from build123d import *

# Parameters (mm, degrees)
F0_R     = 11
F1_DEPTH = 2
F2_R     = 2.5
F3_DEPTH = 25
F4_R     = 11
F4_R_2   = 9
F5_DEPTH = 10


with BuildPart() as f1:
    # F0 (on Front) → F1 (new body)
    with BuildSketch(Plane.XZ):
        Circle(F0_R)
    extrude(amount=F1_DEPTH)

    # F2 (on face) → F3 (cut)
    with BuildSketch(Plane.XZ.offset(2)):
        Circle(F2_R)
    extrude(amount=-F3_DEPTH, mode=Mode.SUBTRACT)

    # F4 (on face) → F5 (join)
    with BuildSketch(Plane.XZ.offset(2)):
        Circle(F4_R)
        Circle(F4_R_2, mode=Mode.SUBTRACT)
    extrude(amount=F5_DEPTH)


solid = f1.part
Source: CAD feature listing. Evaluate the final solid. Frame: model axes, mm. A direction names the side the tool comes from. Coordinates: 2 decimals unless noted, no trailing zeros. Loops run counter-clockwise (first coordinate to the right, second up) from the corner with the lowest first, then second, coordinate; pieces in that order, holes last. Notation, with made-up numbers: (65.5, -28.5) - (112.5, -28.5) arc R33 cw to (112.5, 8.5) - close; hole circle Ø6 at (-37.5, -1.5). An arc over 180 degrees is marked (long way). One line per item, written item: value. Start each with the question number.
1. Mould query, pull axis Z, two halves, no side actions, for faces 3 (the flat face through (-3, 0, 0)), 4 (the cylindrical face through (-2.38, -5.92, -10.74)), 5 (the cylindrical face through (-0.54, -1.01, -2.44)). Classes: pulls with the +Z half, pulls with the -Z half, needs draft (parallel to the pull), parting line crosses it, or undercut.
2. Contact query for flat-ended pins moving along their axis: P1, Ø2, axis at y = -7, z = -3, coming from the -X side; P2, Ø4, axis at y = -8.5, z = -3.5, coming from the +X side; P3, Ø12, axis at x = 7.5, z = 5, coming from the +Y side; P4, Ø4, axis at x = 3, y = -5, coming from the +Z side. Output: stop coordinate, or through.
3. Ray query, L1, parallel to Z at x = 0, y = -10; L2, parallel to Y at x = 6, z = -6.5; L3, parallel to Z at x = 0, y = -1.2. Return the intervals inside material, ascending.
4. Section D-D (x = 3.25). Return the cut outline in (y, z).
5. Section C-C (y = -0.75). Return the cut outline in (x, z), and give its area (3 significant figures).
6. Section A-A (z = 0). Return the cut outline in (x, y), and give its area (3 significant figures).
7. Set-up query: faces 1 (the flat face through (2, -12, -9)), 2 (the flat face through (2, -2, -2)). Return all of +Z, -Z, +X, -X, +Y, -Y with unobstructed straight access to the full face (end or side cutting, diameter ignored); none if empty.
8. Section B-B (x = 0). Return the cut outline in (y, z), and give its area (3 significant figures).
Verdict:
1. face 3: needs draft
1. face 4: parting line crosses it
1. face 5: undercut
2. P1: stops at x = -10.82
2. P2: stops at x = 10.9
2. P3: stops at y = 0
2. P4: stops at z = 10.95
3. L1: z = -11 to -9, 9 to 11
3. L2: y = -2 to 0
3. L3: z = -11 to -2.5, 2.5 to 11
4. outline: (-12, -10.51) - (0, -10.51) - (0, 10.51) - (-12, 10.51) - (-12, 8.39) - (-2, 8.39) - (-2, -8.39) - (-12, -8.39) - close
5. outline: circle Ø22 at (0, 0); hole circle Ø5 at (0, 0)
5. area: 360 mm2
6. outline: (-11, -12) - (-9, -12) - (-9, -2) - (-2.5, -2) - (-2.5, 0) - (-11, 0) - close; (2.5, -2) - (9, -2) - (9, -12) - (11, -12) - (11, 0) - (2.5, 0) - close
6. area: 74.0 mm2
7. face 1: +Z, -Z, +X, -X, -Y
7. face 2: -Y
8. outline: (-12, -11) - (0, -11) - (0, -2.5) - (-2, -2.5) - (-2, -9) - (-12, -9) - close; (-12, 9) - (-2, 9) - (-2, 2.5) - (0, 2.5) - (0, 11) - (-12, 11) - close
8. area: 74.0 mm2
